CAD build for the part. Positions are in the model's coordinates, mm. A direction names the side the tool comes from. Coordinates: 2 decimals unless noted, no trailing zeros. Order: outer loops, then holes, each group sorted by start corner. A loop starts at its lowest first (then second) coordinate and runs counter-clockwise, first axis right, second up.
from build123d import *

# Parameters (mm, degrees)
SKETCH1_W           = 129.9464
SKETCH1_H           = 83.9724
BOSS_EXTRUDE1_DEPTH = 5.7912
SKETCH7_W           = 106.1212
SKETCH7_H           = 82.55
BOSS_EXTRUDE2_DEPTH = 5.7912
SKETCH12_W          = 5.7912
SKETCH12_H          = 27.516666666
CUT_EXTRUDE9_DEPTH  = 141.585631649
SKETCH15_W          = 35.373733334
SKETCH15_H          = 5.7912
CUT_EXTRUDE12_DEPTH = 141.585631649
SKETCH18_R          = 1.397
SKETCH18_W          = 75.438
SKETCH18_H          = 32.512
CUT_EXTRUDE15_DEPTH = 141.585631649
SKETCH19_W          = 19.558
SKETCH19_H          = 2.6035
CUT_EXTRUDE16_DEPTH = 141.585631649
SKETCH20_W          = 2.0828
SKETCH20_H          = 6.1722
CUT_EXTRUDE17_DEPTH = 141.585631649
CAVITY1_START       = 59.182
CAVITY1_OUTLINE_W   = 27.9908
CAVITY1_OUTLINE_H   = 5.7912
CAVITY1_OUTLINE_W_2 = 25.036356667
CAVITY1_OUTLINE_W_3 = 27.516666667
CAVITY1_DEPTH       = 5.7912
CAVITY1_START_2     = -64.9732
CAVITY1_2_OUTLINE_W = 27.9908
CAVITY1_2_OUTLINE_H = 5.7912
CAVITY1_2_DEPTH     = 5.7912
CAVITY1_START_3     = -59.182
CAVITY1_3_OUTLINE_W = 5.7912
CAVITY1_3_OUTLINE_H = 5.7912
CAVITY1_3_DEPTH     = 37.524266667
CAVITY1_START_4     = 21.657733333
CAVITY1_4_OUTLINE_W = 5.7912
CAVITY1_4_OUTLINE_H = 5.7912
CAVITY1_4_DEPTH     = 37.524266667
CAVITY1_START_5     = -45.228933333
CAVITY1_5_OUTLINE_W = 5.7912
CAVITY1_5_OUTLINE_H = 5.7912
CAVITY1_5_DEPTH     = 9.872133333
CAVITY1_6_OUTLINE_W = 5.7912
CAVITY1_6_OUTLINE_H = 5.7912
CAVITY1_6_DEPTH     = 4.080933333
CAVITY1_START_6     = -7.704666667
CAVITY1_7_OUTLINE_W = 5.7912
CAVITY1_7_OUTLINE_H = 5.7912
CAVITY1_7_DEPTH     = 39.234533334
SKETCH21_R          = 2.54
CUT_EXTRUDE18_DEPTH = 141.585631649
SKETCH22_R          = 5.8674
SKETCH22_W          = 10.922
SKETCH22_H          = 12.7
CUT_EXTRUDE19_DEPTH = 141.585631649


# Read off the part's stored shape, not the designer's step: Cavity1
with BuildPart() as part:
    # Sketch1 → Boss-Extrude1 (new body)
    with BuildSketch(Plane.XY):
        Rectangle(SKETCH1_W, SKETCH1_H)
    extrude(amount=BOSS_EXTRUDE1_DEPTH)

    # Sketch7 → Boss-Extrude2 (add)
    with BuildSketch(Plane.XY.offset(5.7912)):
        with Locations((11.9126, 83.2612)):
            Rectangle(SKETCH7_W, SKETCH7_H)
    extrude(amount=-BOSS_EXTRUDE2_DEPTH)

    # Sketch12 → Cut-Extrude9 (cut, through all)
    with BuildSketch(Plane.XY.offset(5.7912)):
        with Locations((-38.2524, 83.2612)):
            Rectangle(SKETCH12_W, SKETCH12_H)
    extrude(amount=-CUT_EXTRUDE9_DEPTH, mode=Mode.SUBTRACT)

    # Sketch15 → Cut-Extrude12 (cut, through all)
    with BuildSketch(Plane.XY.offset(5.7912)):
        with Locations((11.9126, 121.6406)):
            Rectangle(SKETCH15_W, SKETCH15_H)
    extrude(amount=-CUT_EXTRUDE12_DEPTH, mode=Mode.SUBTRACT)

    # Sketch18 → Cut-Extrude15 (cut, through all)
    with BuildSketch(Plane.XY.offset(5.7912)):
        with Locations((-35.183452425, 18.449919855)):
            Circle(SKETCH18_R)
        with Locations((35.276147575, 18.449919855)):
            Circle(SKETCH18_R)
        with Locations(Location((35.276147575, -20.666080145, 0), (0, 0, 180))):
            Circle(SKETCH18_R)
        with Locations(Location((-35.183452425, -20.666080145, 0), (0, 0, 180))):
            Circle(SKETCH18_R)
        with Locations((-0.004452425, -1.108080145)):
            Rectangle(SKETCH18_W, SKETCH18_H)
    extrude(amount=-CUT_EXTRUDE15_DEPTH, mode=Mode.SUBTRACT)

    # Sketch19 → Cut-Extrude16 (cut, through all)
    with BuildSketch(Plane.XY.offset(5.7912)):
        with Locations((55.1942, 43.16476)):
            Rectangle(SKETCH19_W, SKETCH19_H)
    extrude(amount=-CUT_EXTRUDE16_DEPTH, mode=Mode.SUBTRACT)

    # Sketch20 → Cut-Extrude17 (cut, through all)
    with BuildSketch(Plane.XY.offset(5.7912)):
        with Locations((55.1942, 43.16476)):
            Rectangle(SKETCH20_W, SKETCH20_H)
    extrude(amount=-CUT_EXTRUDE17_DEPTH, mode=Mode.SUBTRACT)

    # Cavity1 outline → Cavity1 (cut)
    with BuildSketch(Plane.YZ.offset(CAVITY1_START)):
        with Locations((-27.9908, 2.8956)):
            Rectangle(CAVITY1_OUTLINE_W, CAVITY1_OUTLINE_H)
        with BuildLine():
            Line((13.9954, 5.7912), (13.9954, 0))
            Line((13.9954, 0), (41.86301, 0))
            Line((41.86301, 0), (41.86301, 1.598840513))
            ThreePointArc((41.86301, 1.598840513), (40.447383333, 2.8956), (41.86301, 4.192359487))
            Line((41.86301, 4.192359487), (41.86301, 5.7912))
            Line((41.86301, 5.7912), (13.9954, 5.7912))
        make_face()
        with Locations((56.984688334, 2.8956)):
            Rectangle(CAVITY1_OUTLINE_W_2, CAVITY1_OUTLINE_H)
        with Locations((110.777866667, 2.8956)):
            Rectangle(CAVITY1_OUTLINE_W_3, CAVITY1_OUTLINE_H)
    extrude(amount=CAVITY1_DEPTH, mode=Mode.SUBTRACT)

    # Cavity1 2 outline → Cavity1 2 (cut)
    with BuildSketch(Plane.YZ.offset(CAVITY1_START_2)):
        with Locations((-27.9908, 2.8956)):
            Rectangle(CAVITY1_2_OUTLINE_W, CAVITY1_2_OUTLINE_H)
        with Locations((27.9908, 2.8956)):
            Rectangle(CAVITY1_2_OUTLINE_W, CAVITY1_2_OUTLINE_H)
    extrude(amount=CAVITY1_2_DEPTH, mode=Mode.SUBTRACT)

    # Cavity1 3 outline → Cavity1 3 (cut)
    with BuildSketch(Plane.YZ.offset(CAVITY1_START_3)):
        with Locations((-39.0906, 2.8956)):
            Rectangle(CAVITY1_3_OUTLINE_W, CAVITY1_3_OUTLINE_H)
    extrude(amount=CAVITY1_3_DEPTH, mode=Mode.SUBTRACT)

    # Cavity1 4 outline → Cavity1 4 (cut)
    with BuildSketch(Plane.YZ.offset(CAVITY1_START_4)):
        with Locations((-39.0906, 2.8956)):
            Rectangle(CAVITY1_4_OUTLINE_W, CAVITY1_4_OUTLINE_H)
    extrude(amount=CAVITY1_4_DEPTH, mode=Mode.SUBTRACT)

    # Cavity1 5 outline → Cavity1 5 (cut)
    with BuildSketch(Plane.YZ.offset(CAVITY1_START_5)):
        with Locations((39.0906, 2.8956)):
            Rectangle(CAVITY1_5_OUTLINE_W, CAVITY1_5_OUTLINE_H)
    extrude(amount=CAVITY1_5_DEPTH, mode=Mode.SUBTRACT)

    # Cavity1 6 outline → Cavity1 6 (cut)
    with BuildSketch(Plane.YZ.offset(CAVITY1_START_3)):
        with Locations((39.0906, 2.8956)):
            Rectangle(CAVITY1_6_OUTLINE_W, CAVITY1_6_OUTLINE_H)
    extrude(amount=CAVITY1_6_DEPTH, mode=Mode.SUBTRACT)

    # Cavity1 7 outline → Cavity1 7 (cut)
    with BuildSketch(Plane.YZ.offset(CAVITY1_START_6)):
        with Locations((121.6406, 2.8956)):
            Rectangle(CAVITY1_7_OUTLINE_W, CAVITY1_7_OUTLINE_H)
    extrude(amount=CAVITY1_7_DEPTH, mode=Mode.SUBTRACT)

    # Sketch21 → Cut-Extrude18 (cut, through all)
    with BuildSketch(Plane.XY.offset(5.7912)):
        with Locations((23.919169713, 28.405342819)):
            Circle(SKETCH21_R)
        with Locations((10.918159713, 28.405342819)):
            Circle(SKETCH21_R)
        with Locations((-1.787317277, 28.405342819)):
            Circle(SKETCH21_R)
    extrude(amount=-CUT_EXTRUDE18_DEPTH, mode=Mode.SUBTRACT)

    # Sketch22 → Cut-Extrude19 (cut, through all)
    with BuildSketch(Plane.XY.offset(5.7912)):
        with Locations((27.368980229, 46.405060213)):
            Circle(SKETCH22_R)
        with Locations((-6.74229364, 46.405060213)):
            Circle(SKETCH22_R)
        with Locations((27.368980229, 69.094682683)):
            Circle(SKETCH22_R)
        with Locations((27.368980229, 93.171449402)):
            Circle(SKETCH22_R)
        with Locations((995.334727121, -604.282322998)):
            Rectangle(SKETCH22_W, SKETCH22_H)
        with Locations((995.334727121, -676.824722998)):
            Rectangle(SKETCH22_W, SKETCH22_H)
        with Locations((995.334727121, -628.971122998)):
            Rectangle(SKETCH22_W, SKETCH22_H)
        with Locations((995.334727121, -653.117356371)):
            Rectangle(SKETCH22_W, SKETCH22_H)
    extrude(amount=-CUT_EXTRUDE19_DEPTH, mode=Mode.SUBTRACT)


solid = part.part
1) Slice it at B-B (x = 48). List the corners of the cut face in (y, z) (3 decimals).
2) Slice it at C-C (y = 82). List the corners of the cut face in (x, z).
3) Drill centre lines: probe 1 along Y at (x, z) = (-41, 0.5) (3 decimals); probe 2 along Y at (x, z) = (-5, 3.55) (3 decimals); probe 3 along Y at (x, z) = (23, 3.85) (3 decimals). Where is each one in solid material? Low to high.
4) Which spindle directions (+Z, -Z, +X, -X, +Y, -Y) get a long thin tool onto all of the face, cutting with end or side? Do faces 5 (the flat face through (12, 118.745, 3)), 6 (the flat face through (-21.658, -39, 3)), 7 (the flat face through (-1, 15.148, 3)). Say none if no direction does.
5) Pin check, flat tips, straight feed: P1, Ø3, axis at y = 53.5, z = 2.5, coming from the +X side; P2, Ø0.9, axis at x = 58.5, z = 3.5, coming from the -Y side (3 decimals); P3, Ø3, axis at x = 63.5, z = 3, coming from the -Y side. Stop position of each tip, or through.
6) Slice it at A-A (x = -26.5). List the corners of the cut face in (y, z) (3 decimals), plus the area to 3 significant figures.
7) Two-plate mould, pull along Y, no slides. Class faces 1 (the cylindrical face through (26.097, 63.367, 2.936)), 2 (the flat face through (-35.357, 39, 3)), 3 (the flat face through (-41, -36.195, 3)), 4 (the flat face through (-59.182, -25, 3)): released by +Y, released by -Y, zero draft, split by the parting line, or undercut.
Worked out:
1. outline: (-36.195, 0) - (41.863, 0) - (41.863, 5.791) - (-36.195, 5.791) - close; (44.467, 0) - (124.536, 0) - (124.536, 5.791) - (44.467, 5.791) - close
2. outline: (-35.36, 0) - (64.97, 0) - (64.97, 5.79) - (-35.36, 5.79) - close
3. probe 1: y = -36.195 to 36.195, 41.986 to 69.503, 97.02 to 124.536
3. probe 2: y = -41.986 to -17.364, 15.148 to 40.802, 52.008 to 118.745
3. probe 3: y = -36.195 to -17.364, 15.148 to 26.037, 30.773 to 42.489, 50.321 to 65.178, 73.011 to 89.255, 97.088 to 118.745
4. face 5: +Z, -Z, +Y
4. face 6: +Z, -Z, -X, -Y
4. face 7: +Z, -Z
5. P1: stops at x = 59.18
5. P2: stops at y = -36.195
5. P3: stops at y = -14
6. outline: (-36.195, 0) - (-17.364, 0) - (-17.364, 5.791) - (-36.195, 5.791) - close; (15.148, 0) - (124.536, 0) - (124.536, 5.791) - (15.148, 5.791) - close
6. area: 743 mm2
7. face 1: undercut
7. face 2: undercut
7. face 3: released by -Y
7. face 4: zero draft
